from build123d import *

# Parameters (mm, degrees)
SKETCH1_R                      = 17.5
BOSS_EXTRUDE1_DEPTH            = 3
BOSS_EXTRUDE2_DEPTH            = 8
SKETCH3_R                      = 4
BOSS_EXTRUDE3_DEPTH            = 8
SKETCH4_R                      = 2.2
CUT_EXTRUDE1_DEPTH             = 6
SKETCH5_R                      = 4.2
CUT_EXTRUDE2_DEPTH             = 3.5
CUT_EXTRUDE2_DIRECTION_2_REACH = 28.01


with BuildPart() as part:
    # Sketch1 → Boss-Extrude1 (new, symmetric)
    with BuildSketch(Plane.XY):
        Circle(SKETCH1_R)
    extrude(amount=BOSS_EXTRUDE1_DEPTH, both=True)

    # Sketch2 → Boss-Extrude2 (add)
    with BuildSketch(Plane.XY.offset(3)):
        with BuildLine():
            Line((7.875, 13.63990011), (4.125, 7.144709581))
            ThreePointArc((4.125, 7.144709581), (0, 8.25), (-4.125, 7.144709581))
            Line((-4.125, 7.144709581), (-7.875, 13.63990011))
            ThreePointArc((-7.875, 13.63990011), (0, 15.75), (7.875, 13.63990011))
        make_face()
    extrude(amount=BOSS_EXTRUDE2_DEPTH)

    # Sketch3 → Boss-Extrude3 (add)
    with BuildSketch(Plane.XY.offset(3)):
        Circle(SKETCH3_R)
    extrude(amount=BOSS_EXTRUDE3_DEPTH)

    # Sketch4 → Cut-Extrude1 (cut)
    with BuildSketch(Plane(origin=(0, 0, -3), x_dir=(-1, 0, 0), z_dir=(0, 0, -1))):
        with Locations((-8.485281374, 8.485281374)):
            Circle(SKETCH4_R)
        with Locations((8.485281374, 8.485281374)):
            Circle(SKETCH4_R)
        with Locations((8.485281374, -8.485281374)):
            Circle(SKETCH4_R)
        with Locations((-8.485281374, -8.485281374)):
            Circle(SKETCH4_R)
    extrude(amount=-CUT_EXTRUDE1_DEPTH, mode=Mode.SUBTRACT)

    # Sketch5 → Cut-Extrude2 (cut)
    with BuildSketch(Plane.XY.offset(3)):
        with Locations((-8.485281374, -8.485281374)):
            Circle(SKETCH5_R)
        with Locations(Location((-8.485281374, 8.485281374, 0), (0, 0, 72.312607482))):
            Circle(SKETCH5_R)
        with Locations(Location((8.485281374, 8.485281374, 0), (0, 0, 192.312607482))):
            Circle(SKETCH5_R)
        with Locations((8.485281374, -8.485281374)):
            Circle(SKETCH5_R)
    extrude(amount=-CUT_EXTRUDE2_DEPTH, mode=Mode.SUBTRACT)

    # Cut-Extrude2 direction 2: up to this face of the body (flat: up to its plane)
    cut_extrude2_direction_2_end = Plane(part.part.faces().sort_by_distance((0, 11.8321753, 11))[0])
    # Sketch5 → Cut-Extrude2 direction 2 (cut, up to the picked face)
    with BuildSketch(Plane.XY.offset(3), mode=Mode.PRIVATE) as cut_extrude2_direction_2_sk1:
        with Locations((-8.485281374, -8.485281374)):
            Circle(SKETCH5_R)
    cut_extrude2_direction_2_tool1 = split(extrude(cut_extrude2_direction_2_sk1.sketch, amount=CUT_EXTRUDE2_DIRECTION_2_REACH, mode=Mode.PRIVATE), bisect_by=cut_extrude2_direction_2_end, keep=Keep.BOTH, mode=Mode.PRIVATE)
    # Sketch5 → Cut-Extrude2 direction 2 (cut, up to the picked face)
    with BuildSketch(Plane.XY.offset(3), mode=Mode.PRIVATE) as cut_extrude2_direction_2_sk2:
        with Locations(Location((-8.485281374, 8.485281374, 0), (0, 0, 72.312607482))):
            Circle(SKETCH5_R)
    cut_extrude2_direction_2_tool2 = split(extrude(cut_extrude2_direction_2_sk2.sketch, amount=CUT_EXTRUDE2_DIRECTION_2_REACH, mode=Mode.PRIVATE), bisect_by=cut_extrude2_direction_2_end, keep=Keep.BOTH, mode=Mode.PRIVATE)
    # Sketch5 → Cut-Extrude2 direction 2 (cut, up to the picked face)
    with BuildSketch(Plane.XY.offset(3), mode=Mode.PRIVATE) as cut_extrude2_direction_2_sk3:
        with Locations(Location((8.485281374, 8.485281374, 0), (0, 0, 192.312607482))):
            Circle(SKETCH5_R)
    cut_extrude2_direction_2_tool3 = split(extrude(cut_extrude2_direction_2_sk3.sketch, amount=CUT_EXTRUDE2_DIRECTION_2_REACH, mode=Mode.PRIVATE), bisect_by=cut_extrude2_direction_2_end, keep=Keep.BOTH, mode=Mode.PRIVATE)
    # Sketch5 → Cut-Extrude2 direction 2 (cut, up to the picked face)
    with BuildSketch(Plane.XY.offset(3), mode=Mode.PRIVATE) as cut_extrude2_direction_2_sk4:
        with Locations((8.485281374, -8.485281374)):
            Circle(SKETCH5_R)
    cut_extrude2_direction_2_tool4 = split(extrude(cut_extrude2_direction_2_sk4.sketch, amount=CUT_EXTRUDE2_DIRECTION_2_REACH, mode=Mode.PRIVATE), bisect_by=cut_extrude2_direction_2_end, keep=Keep.BOTH, mode=Mode.PRIVATE)
    add(cut_extrude2_direction_2_tool1.solids().sort_by(Axis((-8.485281, -8.485281, 3), (0, 0, 1)))[0], mode=Mode.SUBTRACT)
    add(cut_extrude2_direction_2_tool2.solids().sort_by(Axis((-8.485281, 8.485281, 3), (0, 0, 1)))[0], mode=Mode.SUBTRACT)
    add(cut_extrude2_direction_2_tool3.solids().sort_by(Axis((8.485281, 8.485281, 3), (0, 0, 1)))[0], mode=Mode.SUBTRACT)
    add(cut_extrude2_direction_2_tool4.solids().sort_by(Axis((8.485281, -8.485281, 3), (0, 0, 1)))[0], mode=Mode.SUBTRACT)


solid = part.part
Here's how the part is built. I have some questions about the finished solid (model axes, mm). A direction names the side the tool comes from. Round coordinates to 2 decimals unless told otherwise and drop trailing zeros. Write each loop counter-clockwise with the first axis right and the second up, starting at its lowest first coordinate (ties: lowest second). Pieces come first, ordered by that corner, then holes.
1. Suppose I cut it at D-D (x = -10). List the corners of the cut face in (y, z) for me.
2. Suppose I cut it at C-C (x = 0). List the corners of the cut face in (y, z) for me, and give its area (3 significant figures).
3. For faces 4 (the cylindrical face through (-6.23, -4.94, 1.27)), 5 (the cylindrical face through (8.772, 10.667, -1.768)), 6 (the flat face through (-7.54, 13.06, 6.94)), 7 (the flat face through (7.547, 13.071, 6.944)), which set-ups out of +Z, -Z, +X, -X, +Y, -Y let a thin tool reach every point of the face, with its end or its side?
4. I need wall thicknesses on L1, parallel to Y at x = 0, z = 7.5; L2, parallel to X at y = 7, z = -1; L3, parallel to X at y = 9, z = -1.25. Which ranges of each line are inside material? Lowest first, please.
5. Suppose I cut it at A-A (z = 9.75). List the corners of the cut face in (x, y) for me (3 decimals), and give its area (3 significant figures).
6. Will these pins go through, and if not, where does the flat tip stop? pin 1 Ø13.5 at (x, y) = (8.49, 8.49) entering from +Z; pin 2 Ø4 at (x, z) = (-7.5, 6) entering from -Y; pin 3 Ø5 at (x, y) = (-8.49, 8.49) entering from +Z; pin 4 Ø2.5 at (x, y) = (8.49, -8.49) entering from -Z.
7. Suppose I cut it at B-B (y = -7). List the corners of the cut face in (x, z) for me.
8. If we mould it in two halves opening along Y, with no side actions, what happens to faces 1 (the flat face through (6, 10, -0.5)), 2 (the flat face through (0, 0, 11)), 3 (the cylindrical face through (-0.12, 15.75, 6.94))? For each: released by +Y, released by -Y, zero draft, split by the parting line, or undercut.
Answer sheet:
1. outline: (-14.36, -3) - (-10.08, -3) - (-10.08, -0.5) - (-12.4, -0.5) - (-12.4, 3) - (-14.36, 3) - close; (-6.89, -3) - (6.89, -3) - (6.89, -0.5) - (4.57, -0.5) - (4.57, 3) - (-4.57, 3) - (-4.57, -0.5) - (-6.89, -0.5) - close; (10.08, -3) - (14.36, -3) - (14.36, 3) - (12.4, 3) - (12.4, -0.5) - (10.08, -0.5) - close
2. outline: (-17.5, -3) - (17.5, -3) - (17.5, 3) - (15.75, 3) - (15.75, 11) - (8.25, 11) - (8.25, 3) - (4, 3) - (4, 11) - (-4, 11) - (-4, 3) - (-17.5, 3) - close
2. area: 334 mm2
3. face 4: +Z
3. face 5: +Z, -Z
3. face 6: +Z, -X, -Y
3. face 7: +Z, +X, -Y
4. L1: y = -4 to 4, 8.25 to 15.75
4. L2: x = -16.04 to -10.11, -6.86 to 6.86, 10.11 to 16.04
4. L3: x = -15.01 to -10.62, -6.35 to 6.35, 10.62 to 15.01
5. outline: (-7.875, 13.64) - (-7.209, 12.487) arc R4.2 cw to (-4.382, 7.59) - (-4.125, 7.145) arc R8.25 cw to (4.125, 7.145) - (4.382, 7.59) arc R4.2 cw to (7.209, 12.487) - (7.875, 13.64) arc R15.75 ccw to start; circle Ø8 at (0, 0)
5. area: 136 mm2
6. pin 1: stops at z = 11
6. pin 2: stops at y = 11.44
6. pin 3: stops at z = -0.5
6. pin 4: passes through
7. outline: (-16.04, -3) - (-10.11, -3) - (-10.11, -0.5) - (-12.41, -0.5) - (-12.41, 3) - (-16.04, 3) - close; (-6.86, -3) - (6.86, -3) - (6.86, -0.5) - (4.56, -0.5) - (4.56, 3) - (-4.56, 3) - (-4.56, -0.5) - (-6.86, -0.5) - close; (10.11, -3) - (16.04, -3) - (16.04, 3) - (12.41, 3) - (12.41, -0.5) - (10.11, -0.5) - close
8. face 1: undercut
8. face 2: zero draft
8. face 3: released by +Y
